from build123d import *

# Parameters (mm, degrees)
F0_W      = 194
F0_H      = 194
F0_R      = 70
F1_DEPTH  = 2
F0_R_2    = 1.5
F2_DEPTH  = 5
F0_W_2    = 3
F0_H_2    = 20
F3_DEPTH  = 10
F5_DEPTH  = 3
F7_DEPTH  = 3
F8_R      = 1.25
F9_DEPTH  = 4
F11_R     = 1.25
F12_DEPTH = 4
F14_DEPTH = 3
F15_W     = 20
F15_H     = 4
F16_DEPTH = 2
F17_W     = 20
F17_H     = 4
F18_DEPTH = 2


with BuildPart() as f1:
    # F0 (on Top) → F1 (new body)
    with BuildSketch(Plane.XY):
        Rectangle(F0_W, F0_H)
        Circle(F0_R, mode=Mode.SUBTRACT)
    extrude(amount=F1_DEPTH)



with BuildPart() as f2:
    # F0 (on Top) → F2 (new body)
    with BuildSketch(Plane.XY):
        with BuildLine():
            Line((-7.5, 99), (7.5, 99))
            Line((7.5, 99), (7.5, 109.5))
            ThreePointArc((7.5, 109.5), (0, 117), (-7.5, 109.5))
            Line((-7.5, 109.5), (-7.5, 99))
        make_face()
        with Locations((0, 109.5)):
            Circle(F0_R_2, mode=Mode.SUBTRACT)
    extrude(amount=F2_DEPTH)


with BuildPart() as f1_1:
    add(f1.part)

    add(f2.part)  # F3 merges F2
    # F0 (on Top) → F3 (join)
    with BuildSketch(Plane.XY):
        Polygon((96, -99), (99, -99), (99, 99), (7.5, 99), (-7.5, 99), (-99, 99), (-99, -99), (-96, -99), align=None)
        Rectangle(F0_W, F0_H, mode=Mode.SUBTRACT)
        with Locations((-97.5, -109)):
            Rectangle(F0_W_2, F0_H_2)
        with Locations((97.5, -109)):
            Rectangle(F0_W_2, F0_H_2)
    extrude(amount=F3_DEPTH)

    # F4 (on face) → F5 (join)
    with BuildSketch(Plane.YZ.offset(-96)):
        with BuildLine():
            Line((-119, 0), (-119, 10))
            ThreePointArc((-119, 10), (-124, 5), (-119, 0))
        make_face()
    extrude(amount=-F5_DEPTH)

    # F6 (on face) → F7 (join)
    with BuildSketch(Plane.YZ.offset(99)):
        with BuildLine():
            Line((-119, 0), (-119, 10))
            ThreePointArc((-119, 10), (-124, 5), (-119, 0))
        make_face()
    extrude(amount=-F7_DEPTH)

    # F8 (on face) → F9 (join)
    with BuildSketch(Plane.YZ.offset(-96)):
        with Locations((-119, 5)):
            Circle(F8_R)
    extrude(amount=F9_DEPTH)

    # F11 (on offset) → F12 (join)
    with BuildSketch(Plane(origin=(96, 0, 0), x_dir=(0, -1, 0), z_dir=(-1, 0, 0))):
        with Locations((119, 5)):
            Circle(F11_R)
    extrude(amount=F12_DEPTH)

    # F13 (on face) → F14 (join)
    with BuildSketch(Plane.XY.offset(10)):
        with BuildLine():
            Line((-99, 55), (-99, 95))
            Line((-99, 95), (-114, 95))
            ThreePointArc((-114, 95), (-117.5355339059, 93.5355339059), (-119, 90))
            Line((-119, 90), (-119, 60))
            ThreePointArc((-119, 60), (-117.5355339059, 56.4644660941), (-114, 55))
            Line((-114, 55), (-99, 55))
        make_face()
        with BuildLine():
            Line((114, 95), (99, 95))
            Line((99, 95), (99, 55))
            Line((99, 55), (114, 55))
            ThreePointArc((114, 55), (117.5355339059, 56.4644660941), (119, 60))
            Line((119, 60), (119, 90))
            ThreePointArc((119, 90), (117.5355339059, 93.5355339059), (114, 95))
        make_face()
    extrude(amount=-F14_DEPTH)

    # F15 (on face) → F16 (cut, through all)
    with BuildSketch(Plane.YZ.offset(-97)):
        with Locations((-50, 4)):
            Rectangle(F15_W, F15_H)
        with Locations((50, 4)):
            Rectangle(F15_W, F15_H)
    extrude(amount=-F16_DEPTH, mode=Mode.SUBTRACT)

    # F17 (on face) → F18 (cut, through all)
    with BuildSketch(Plane(origin=(97, 0, 0), x_dir=(0, -1, 0), z_dir=(-1, 0, 0))):
        with Locations((50, 4)):
            Rectangle(F17_W, F17_H)
        with Locations((-50, 4)):
            Rectangle(F17_W, F17_H)
    extrude(amount=-F18_DEPTH, mode=Mode.SUBTRACT)


solid = f1_1.part
Work out the finished part from the listing and answer in its coordinate system (mm). A direction names the side the tool comes from. Give positions to 0.01 mm unless a question says otherwise; leave off trailing zeros. Loops run counter-clockwise (first coordinate to the right, second up) from the corner with the lowest first, then second, coordinate; pieces in that order, holes last. Notation, with made-up numbers: (65.25, 69) - (89.25, 69) arc R12 cw to (89.25, 86) - close; hole circle Ø3 at (33, -19). An arc over 180 degrees is marked (long way). Answer in a Markdown table with one row per item.
(1) For a pull along X with two mould halves and no side action, classify faces 4 (the face through (-1, -97, 6)), 5 (the face through (97, -1, 6)), 6 (the face through (1, 99, 6)), 7 (the face through (0, 117, 2)) as pulls with the +X half, pulls with the -X half, needs draft (parallel to the pull), parting line crosses it, or undercut.
Results list:
| item | result |
|---|---|
| face 4 | undercut |
| face 5 | undercut |
| face 6 | needs draft |
| face 7 | parting line crosses it |
(2) Section D-D (y = 87) is taken. Give the vertices of the cut face in (x, z), and give its area (3 significant figures).
Results list:
| item | result |
|---|---|
| outline | (-119, 7) - (-99, 7) - (-99, 0) - (99, 0) - (99, 7) - (119, 7) - (119, 10) - (97, 10) - (97, 2) - (-97, 2) - (-97, 10) - (-119, 10) - close |
| area | 548 mm² |
(3) Section B-B (x = 16.5) is taken. Give the vertices of the cut face in (y, z).
Results list:
| item | result |
|---|---|
| outline | (-99, 0) - (-68.03, 0) - (-68.03, 2) - (-97, 2) - (-97, 10) - (-99, 10) - close; (68.03, 0) - (99, 0) - (99, 10) - (97, 10) - (97, 2) - (68.03, 2) - close |
(4) Section A-A (y = 0) is taken. Give the vertices of the cut face in (x, z), and give its area (3 significant figures).
Results list:
| item | result |
|---|---|
| outline | (-99, 0) - (-70, 0) - (-70, 2) - (-97, 2) - (-97, 10) - (-99, 10) - close; (70, 0) - (99, 0) - (99, 10) - (97, 10) - (97, 2) - (70, 2) - close |
| area | 148 mm² |
(5) Consider L1, parallel to Y at x = 0, z = 1.5; L2, parallel to Y at x = -9.5, z = 7.5. Determine where each line is inside the solid, lowest interval first. Write a range as [from, to].
Results list:
| item | result |
|---|---|
| L1 | y = [-99, -70], [70, 108], [111, 117] |
| L2 | y = [-99, -97], [97, 99] |
(6) A tool of negligible diameter and unlimited length cuts with its end or side. For faces 1 (the face through (0, 106, 5)), 2 (the face through (-1, 97, 6)), 3 (the face through (-109, 75, 7)), from which of +Z, -Z, +X, -X, +Y, -Y can it reach the whole face along a straight path? Write none if from no direction.
Results list:
| item | result |
|---|---|
| face 1 | +Z, +X, -X, +Y |
| face 2 | +Z |
| face 3 | -Z, -X, +Y, -Y |
(7) Flat-ended cylindrical pins translate along their axes: pin 1 Ø6 at (y, z) = (87.5, 1) entering from +X; pin 2 Ø2.5 at (x, z) = (106, 8.5) entering from -Y; pin 3 Ø1 at (x, z) = (97.5, 3) entering from -Y. Find the tip coordinate at first contact, or state that the pin passes through.
Results list:
| item | result |
|---|---|
| pin 1 | stops at x = 99 |
| pin 2 | stops at y = 55 |
| pin 3 | stops at y = -123.77 |
(8) Section C-C (x = -86.5) is taken. Give the vertices of the cut face in (y, z), and give its area (3 significant figures).
Results list:
| item | result |
|---|---|
| outline | (-99, 0) - (99, 0) - (99, 10) - (97, 10) - (97, 2) - (-97, 2) - (-97, 10) - (-99, 10) - close |
| area | 428 mm² |
